Could you check a few things on this model? Use its own coordinates, in mm. Face numbers are marked on the shaded views. A direction names the side the tool comes from. Give positions to 0.01 mm unless a question says otherwise; leave off trailing zeros. Answer as CSV lines item,"result". Start each with the question number.
(1) On a 3-axis mill with a long thin cutter (end or side, diameter ignored), from which of +Z, -Z, +X, -X, +Y, -Y can I reach the whole of each face in a straight line? I mean the marked faces 5 and 6. Say none if no direction works.
(2) Will these pins go through, and if not, where does the flat tip stop? pin 1 Ø1.5 at (x, z) = (-13, -10.5) entering from +Y; pin 2 Ø4 at (x, y) = (-14, -117.5) entering from +Z; pin 3 Ø5 at (x, y) = (-0.5, -84) entering from +Z.
(3) I want a section at A-A (y = -59). Give the number of separate pieces and of enclosed holes in the cut face, plus the area to 3 significant figures.
(4) We'd pull the mould along Z, two halves only. Please class the marked faces 1, 2, 3 and 4: released by +Z, released by -Z, zero draft, split by the parting line, or undercut.
(5) I need wall thicknesses on L1, parallel to X at y = -104, z = -2; L2, parallel to Z at x = 13, y = -72.5; L3, parallel to Z at x = 1, y = -72.5. Which ranges of each line are inside material? Lowest first, please.
```python
from build123d import *

# Parameters (mm, degrees)
F0_W      = 60
F0_H      = 40
F0_W_2    = 50
F0_H_2    = 32.5
F1_DEPTH  = 140
F2_T      = -0.5
F4_DEPTH  = 40
F6_DEPTH  = 60
F7_DEPTH  = 140
F8_W      = 10
F8_H      = 40
F9_DEPTH  = 60
F11_DEPTH = 60
F12_DEPTH = 60


with BuildPart() as f1:
    # F0 (on Front) → F1 (new body)
    with BuildSketch(Plane.XZ):
        Rectangle(F0_W, F0_H)
        Rectangle(F0_W_2, F0_H_2, mode=Mode.SUBTRACT)
    extrude(amount=F1_DEPTH)

    # F2 (hollow: no face is removed)
    offset(amount=F2_T, kind=Kind.INTERSECTION, mode=Mode.SUBTRACT)

    # F3 (on face) → F4 (join, through all)
    with BuildSketch(Plane.XY.offset(20)):
        Polygon((-29.8089313839, -140), (0, -70.5899032727), (-0.1578061569, -70.2224516363), (-30, -139.71), (-30, -140), align=None)
        Polygon((30, -139.71), (0.1578061569, -70.2224516363), (0, -70.5899032727), (29.8089313839, -140), (30, -140), align=None)
        Polygon((-0.1578061569, -70.2224516363), (0, -69.855), (-30, 0), (-30, -0.3179561596), (-30, -0.7349032727), align=None)
        Polygon((0, -70.5899032727), (0.1578061569, -70.2224516363), (0, -69.855), (-0.1578061569, -70.2224516363), align=None)
        Polygon((0.1578061569, -70.2224516363), (30, -0.7349032727), (30, 0), (0, -69.855), align=None)
    extrude(amount=-F4_DEPTH)

    # F5 (on face) → F6 (join, through all)
    with BuildSketch(Plane.YZ.offset(30)):
        Polygon((-69.472192033, 0.1508022763), (-70, 0), (-69.472192033, -0.1508022763), (-68.9443840661, 0), align=None)
        Polygon((0, 20), (-69.472192033, 0.1508022763), (-68.9443840661, 0), (0, 19.6983954474), align=None)
        Polygon((-68.9443840661, 0), (-69.472192033, -0.1508022763), (0, -20), (0, -19.6983954474), align=None)
        Polygon((-140, 20), (-70, 0), (-69.472192033, 0.1508022763), (-138.9443840661, 20), align=None)
        Polygon((-70, 0), (-140, -20), (-138.9443840661, -20), (-69.472192033, -0.1508022763), align=None)
    extrude(amount=-F6_DEPTH)

    # F0 (on Front) → F7 (cut)
    with BuildSketch(Plane.XZ):
        Rectangle(F0_W_2, F0_H_2)
    extrude(amount=F7_DEPTH, mode=Mode.SUBTRACT)

    # F8 (on face) → F9 (join, through all)
    with BuildSketch(Plane.YZ.offset(30)):
        with Locations((-135, 0)):
            Rectangle(F8_W, F8_H)
    extrude(amount=-F9_DEPTH)

    # F10 (on face) → F11 (cut, through all)
    with BuildSketch(Plane(origin=(-30, 0, 0), x_dir=(0, -1, 0), z_dir=(-1, 0, 0))):
        Polygon((83.6813354429, -20), (140, -20), (140, -16.54), align=None)
        Polygon((83.6813354429, 20), (140, 16.54), (140, 20), align=None)
    extrude(amount=-F11_DEPTH, mode=Mode.SUBTRACT)

    # F10 (on face) → F12 (join, through all)
    with BuildSketch(Plane(origin=(-30, 0, 0), x_dir=(0, -1, 0), z_dir=(-1, 0, 0))):
        Polygon((78.9609849453, 20), (140, 16.25), (140, 16.54), (83.6813354429, 20), align=None)
        Polygon((83.6813354429, -20), (140, -16.54), (140, -16.25), (78.9609849453, -20), align=None)
    extrude(amount=-F12_DEPTH)


solid = f1.part
```
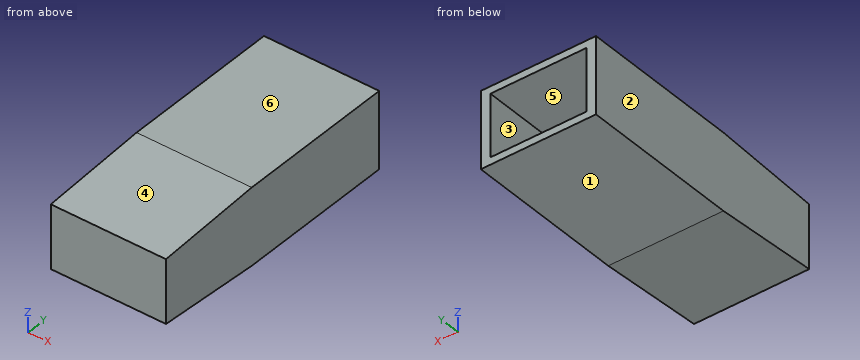
Final values:
1,face 5,"+Y"
1,face 6,"+Z, +X, -X, +Y, -Y"
2,pin 1,"y = -130"
2,pin 2,"z = 18.05"
2,pin 3,"z = 20"
3,separate pieces,"1"
3,enclosed holes,"9"
3,area,"191 mm²"
4,face 1,"released by -Z"
4,face 2,"zero draft"
4,face 3,"undercut"
4,face 4,"released by +Z"
5,L1,"-30 to -29.5, -25.5 to -25, 25 to 25.5, 29.5 to 30"
5,L2,"-20 to -19.5, -16.75 to -16.25, 16.25 to 16.75, 19.5 to 20"
5,L3,"-20 to -16.25, 16.25 to 20"
